```python
from build123d import *

# Parameters (mm, degrees)
CUT_EXTRUDE1_DEPTH      = 59.855755878
CUT_EXTRUDE1_DEPTH_BACK = 59.855755878
SKETCH2_R               = 3.253242351
SKETCH2_R_2             = 3.475880092
SKETCH2_R_3             = 3.633937036


with BuildPart() as part:
    # Sketch1 → Revolve2 (revolve)
    with BuildSketch(Plane.XY, mode=Mode.PRIVATE) as revolve2_sk:
        Polygon((20, 12), (20, 15), (4, 20), (4, 33), (13, 35), (13, 38), (-13, 38), (-13, 35), (-4, 33), (-4, 20), (-20, 15), (-20, 12), align=None)
    revolve(revolve2_sk.sketch.rotate(Axis((29.536406987, 0, 0), (-1, 0, 0)), 90), axis=Axis((29.536406987, 0, 0), (-1, 0, 0)))

    # Sketch2 → Cut-Extrude1 (cut, two sides: drawn at the far end of the back side and taken through both)
    with BuildSketch(Plane(origin=(4, 0, 0), x_dir=(0, 0, -1), z_dir=(1, 0, 0)).offset(-CUT_EXTRUDE1_DEPTH_BACK)):
        with Locations((-21.868025182, 9.381578111)):
            Circle(SKETCH2_R)
        with Locations((4.169252075, 24.089721188)):
            Circle(SKETCH2_R_2)
        with Locations((21.558463792, 12.634820462)):
            Circle(SKETCH2_R_3)
    extrude(amount=CUT_EXTRUDE1_DEPTH + CUT_EXTRUDE1_DEPTH_BACK, mode=Mode.SUBTRACT)


solid = part.part
```
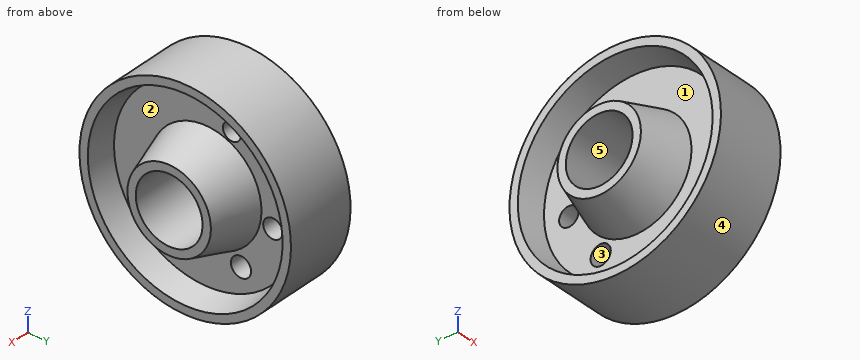
For this review, take the finished solid that the model builds, in its own axes (mm). Face numbers are marked on the shaded views. A direction names the side the tool comes from. Coordinates: 2 decimals unless noted, no trailing zeros. Order: outer loops, then holes, each group sorted by start corner. A loop starts at its lowest first (then second) coordinate and runs counter-clockwise, first axis right, second up. Notation, with made-up numbers: (-25, 20.25) - (13, 20.25) arc R7 ccw to (13, 29.25) - close; hole circle Ø9 at (37, -12.5). An arc over 180 degrees is marked (long way). Answer as a JSON object with one key per item and string values. Group by question number.
1. Clearance check with flat-ended pins moving along their axes: P1, Ø5, axis at x = -15, y = 6, coming from the -Z side; P2, Ø4, axis at x = -10, z = 27.5, coming from the -Y side; P3, Ø3, axis at x = -6.5, y = 1.5, coming from the +Z side; P4, Ø8, axis at y = -8.5, z = 26, coming from the +X side. State where each tip first meets the part, or that it passes through.
2. For probe 1 along Y at (x, z) = (-11.5, -14.5); probe 2 along Y at (x, z) = (9, 0); probe 3 along Y at (x, z) = (-8, 2.5), list the stretches that pass through material, from the lowest coordinate up.
3. The part is to be moulded in two halves that separate along Z. For the marked faces 4 and 5, say which applies: pulls with the +Z half, pulls with the -Z half, needs draft (parallel to the pull), parting line crosses it, or undercut.
4. We need section B-B on z = -6.5. Give the number of separate pieces and of enclosed holes in the cut face, then the cut area to 3 significant figures.
5. We need section D-D on x = 17. State the section outline as (y, z) points (1 decimal).
6. We need section C-C on x = -14. State the section outline as (y, z) points (3 decimals), then the cut area to 3 significant figures.
7. For the marked faces 1, 2 and 3, list the 3-axis set-ups (+Z, -Z, +X, -X, +Y, -Y) from which the entire face can be reached by the end or side of a thin tool; tool diameter is ignored.
8. We need section A-A on y = 0. State the section outline as (x, z) points, then the cut area to 3 significant figures.
Final values:
{
 "1": {"P1": "z = -37.73", "P2": "y = -28.17", "P3": "z = 38", "P4": "x = 4"},
 "2": {"probe 1": "-35.12 to -31.49, -10.07 to 10.07, 31.49 to 35.12", "probe 2": "-38 to -34.11, -18.44 to -12, 12 to 18.44, 34.11 to 38", "probe 3": "-37.92 to -33.8, -18.58 to -11.74, 11.74 to 18.58, 33.8 to 37.92"},
 "3": {"face 4": "parting line crosses it", "face 5": "undercut"},
 "4": {"separate pieces": "3", "enclosed holes": "0", "area": "936 mm²"},
 "5": {"outline": "circle Ø31.9 at (0, 0); hole circle Ø24 at (0, 0)"},
 "6": {"outline": "circle Ø33.75 at (0, 0); hole circle Ø24 at (0, 0)", "area": "442 mm²"},
 "7": {"face 1": "-X", "face 2": "+X", "face 3": "+X, -X"},
 "8": {"outline": "(-20, -15) - (-4, -20) - (-4, -33) - (-13, -35) - (-13, -38) - (13, -38) - (13, -35) - (4, -33) - (4, -20) - (20, -15) - (20, -12) - (-20, -12) - close; (-20, 12) - (20, 12) - (20, 15) - (4, 20) - (4, 33) - (13, 35) - (13, 38) - (-13, 38) - (-13, 35) - (-4, 33) - (-4, 20) - (-20, 15) - close", "area": "912 mm²"}
}
